from build123d import *

# Parameters (mm, degrees)
SKETCH1_R           = 26.9875
BOSS_EXTRUDE1_DEPTH = 562.356
SKETCH2_R           = 22.86
BOSS_EXTRUDE2_DEPTH = 2.54
SKETCH3_R           = 13.915766971
BOSS_EXTRUDE3_DEPTH = 5.08
SKETCH4_R           = 16.731786723
BOSS_EXTRUDE4_DEPTH = 7.62
FILLET1_R           = 0.508
FILLET2_R           = 0.508
FILLET3_R           = 0.508
FILLET4_R           = 1.27
SKETCH5_R           = 23.627835933
BOSS_EXTRUDE5_DEPTH = 2.54
SKETCH6_R           = 28.8925
BOSS_EXTRUDE6_DEPTH = 9.525
SKETCH7_R           = 15.875
BOSS_EXTRUDE7_DEPTH = 13.208


with BuildPart() as part:
    # Sketch1 → Boss-Extrude1 (new body)
    with BuildSketch(Plane.XY):
        Circle(SKETCH1_R)
    extrude(amount=BOSS_EXTRUDE1_DEPTH)

    # Sketch2 → Boss-Extrude2 (add)
    with BuildSketch(Plane.XY.offset(562.356)):
        Circle(SKETCH2_R)
    extrude(amount=BOSS_EXTRUDE2_DEPTH)

    # Sketch3 → Boss-Extrude3 (add)
    with BuildSketch(Plane.XY.offset(564.896)):
        Circle(SKETCH3_R)
    extrude(amount=BOSS_EXTRUDE3_DEPTH)

    # Sketch4 → Boss-Extrude4 (add)
    with BuildSketch(Plane.XY.offset(569.976)):
        with Locations(Location((0, 0, 0), (0, 0, 180))):
            Circle(SKETCH4_R)
    extrude(amount=BOSS_EXTRUDE4_DEPTH)

    # Fillet1
    fillet1_edges = [part.edges().sort_by_distance(p)[0] for p in [
        (16.731786723, 0, 577.596),
    ]]
    fillet(fillet1_edges, radius=FILLET1_R)

    # Fillet2
    fillet2_edges = [part.edges().sort_by_distance(p)[0] for p in [
        (-13.915766971, 0, 564.896),
    ]]
    fillet(fillet2_edges, radius=FILLET2_R)

    # Fillet3
    fillet3_edges = [part.edges().sort_by_distance(p)[0] for p in [
        (-22.86, 0, 564.896),
    ]]
    fillet(fillet3_edges, radius=FILLET3_R)

    # Fillet4
    fillet4_edges = [part.edges().sort_by_distance(p)[0] for p in [
        (-26.9875, 0, 562.356),
    ]]
    fillet(fillet4_edges, radius=FILLET4_R)

    # Sketch5 → Boss-Extrude5 (add)
    with BuildSketch(Plane(origin=(0, 0, 0), x_dir=(-1, 0, 0), z_dir=(0, 0, -1))):
        Circle(SKETCH5_R)
    extrude(amount=BOSS_EXTRUDE5_DEPTH)

    # Sketch6 → Boss-Extrude6 (add)
    with BuildSketch(Plane(origin=(0, 0, -2.54), x_dir=(-1, 0, 0), z_dir=(0, 0, -1))):
        with Locations(Location((0, 0, 0), (0, 0, 180))):
            Circle(SKETCH6_R)
    extrude(amount=BOSS_EXTRUDE6_DEPTH)

    # Sketch7 → Boss-Extrude7 (add)
    with BuildSketch(Plane(origin=(0, 0, -12.065), x_dir=(-1, 0, 0), z_dir=(0, 0, -1))):
        with Locations(Location((0, 0, 0), (0, 0, 180))):
            Circle(SKETCH7_R)
    extrude(amount=BOSS_EXTRUDE7_DEPTH)


solid = part.part
Input: part model. Units: mm. Frame: model coordinates. A direction names the side the tool comes from. Give positions to 0.01 mm unless a question says otherwise; leave off trailing zeros. Write each loop counter-clockwise with the first axis right and the second up, starting at its lowest first coordinate (ties: lowest second). Pieces come first, ordered by that corner, then holes. Notation, with made-up numbers: M 21,30.5 L 59,30.5 A26 cw 59,49.5 Z; hole C 46.25,-35.75 d8. An arc over 180 degrees is marked long. Use one line per item in the form item = value.
1. Cut plane A-A on z = 425. Return loops of the section in (x, y) (1 decimal).
Outcome:
outline = C 0,0 d54
2. Mould query, pull axis Z, two halves, no side actions, for faces 1 (the face through (0, 0, -25.273)), 2 (the face through (0, -15, 564.896)), 3 (the face through (3.627, 16.334, 573.482)). Classes: released by +Z, released by -Z, zero draft, split by the parting line, or undercut.
Outcome:
face_1 = released by -Z
face_2 = undercut
face_3 = zero draft
3. First-contact query: P1, Ø2, axis at x = 16, z = 398.5, coming from the +Y side; P2, Ø2, axis at x = 15.5, y = -17.5, coming from the +Z side; P3, Ø8, axis at y = 22.5, z = 223.5, coming from the +X side. Flat tips, straight axial feed; report the tip coordinate or a pass-through.
Outcome:
P1 = 22.43
P2 = 564.9
P3 = 19.65
4. Reachability of faces 4 (the face through (-19.89, 18.24, 276.62)), 5 (the face through (12, 12, -12.065)), 6 (the face through (-24, 0, -2.54)) from +Z, -Z, +X, -X, +Y, -Y: full face, straight path, thin tool, end or side. Return the list, or none.
Outcome:
face_4 = +Z
face_5 = -Z
face_6 = none
5. Ray query, L1, parallel to Z at x = -11, y = 9.5; L2, parallel to X at y = -8, z = 543; L3, parallel to Z at x = 8.5, y = 18 (3 decimals). Return the intervals inside material, ascending.
Outcome:
L1 = -25.27 to 564.9, 569.98 to 577.6
L2 = -25.77 to 25.77
L3 = -12.065 to 564.896
